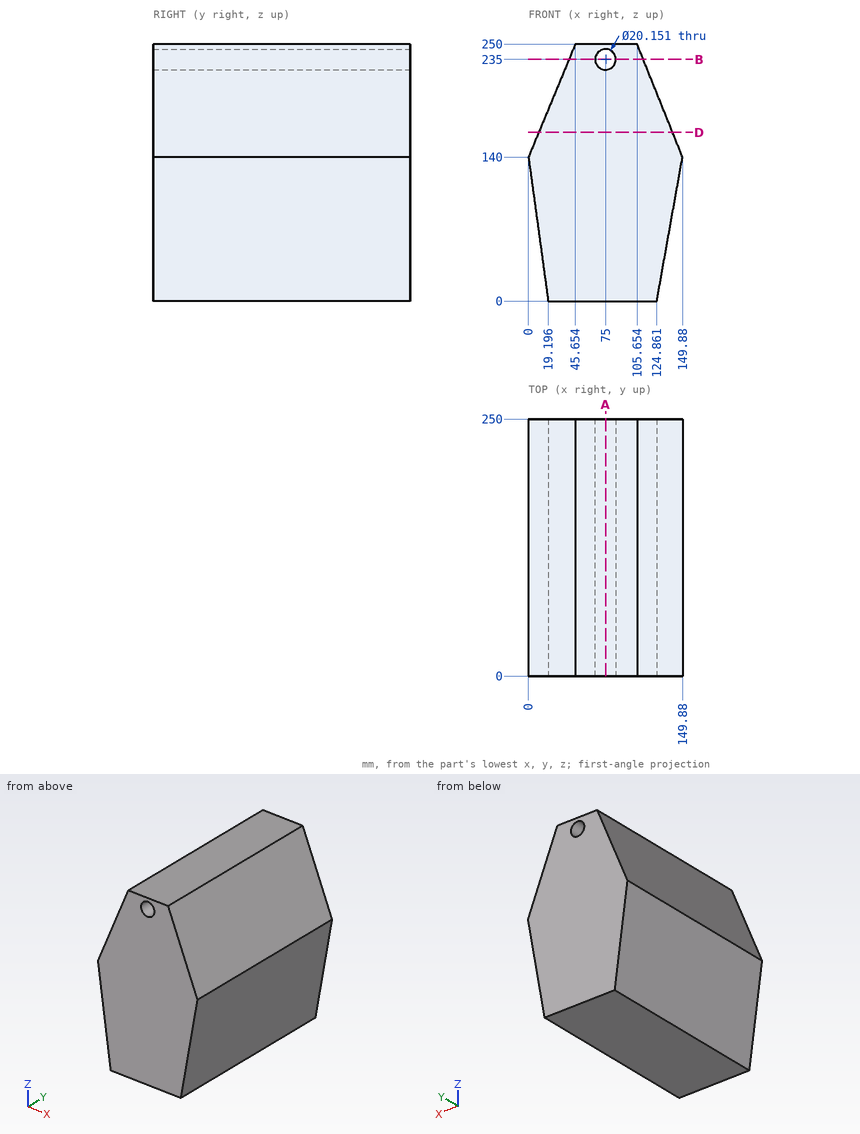
Study the drawing (mm; zero at the part's minimum x, y, z) and answer. Give positions to 0.01 mm unless a question says otherwise; leave off trailing zeros. Write each loop counter-clockwise with the first axis right and the second up, starting at its lowest first coordinate (ties: lowest second). Pieces come first, ordered by that corner, then holes. Notation, with made-up numbers: (83, -10.75) - (118, -10.75) arc R20 ccw to (118, -2.75) - close; hole circle Ø5 at (70, 69.25). An arc over 180 degrees is marked (long way). Write item = value, one per line. Start each with the question number.
Item 1: Each of these flat-tipped pins is pushed along its axis until it touches: P1, Ø1, axis at x = 125, y = 144, coming from the +Z side (1 decimal); P2, Ø3, axis at y = 40.5, z = 109, coming from the -X side (1 decimal); P3, Ø8, axis at x = 34, y = 204, coming from the -Z side; P4, Ø4, axis at x = 19, y = 130, coming from the +Z side (1 decimal). Where does it stop, or does it pass through?
Item 2: Find section B-B (z = 235). Give the vertices of the cut face in (x, y) (1 decimal).
Item 3: Find section A-A (x = 75). Give the vertices of the cut face in (y, z) (1 decimal).
Item 4: Find the intervals of material crossed by probe 1 along Z at (x, y) = (75, 126) (1 decimal); probe 2 along Z at (x, y) = (43.5, 57.5) (1 decimal); probe 3 along X at (y, z) = (143, 19), in increasing order. Write a range as [from, to].
Item 5: Find section D-D (z = 164). Give the vertices of the cut face in (x, y), then the cut area to 3 significant figures.
Response:
q1.P1 = 203.1
q1.P2 = 4
q1.P3 = 0
q1.P4 = 190.6
q2.outline = (39.4, 0) - (64.9, 0) - (64.9, 250) - (39.4, 250) - close; (85.1, 0) - (111.7, 0) - (111.7, 250) - (85.1, 250) - close
q3.outline = (0, 0) - (250, 0) - (250, 224.9) - (0, 224.9) - close; (0, 245.1) - (250, 245.1) - (250, 250) - (0, 250) - close
q4.probe_1 = [0, 224.9], [245.1, 250]
q4.probe_2 = [0, 244.8]
q4.probe_3 = [16.59, 128.26]
q5.outline = (9.96, 0) - (140.23, 0) - (140.23, 250) - (9.96, 250) - close
q5.area = 32,600 mm²
